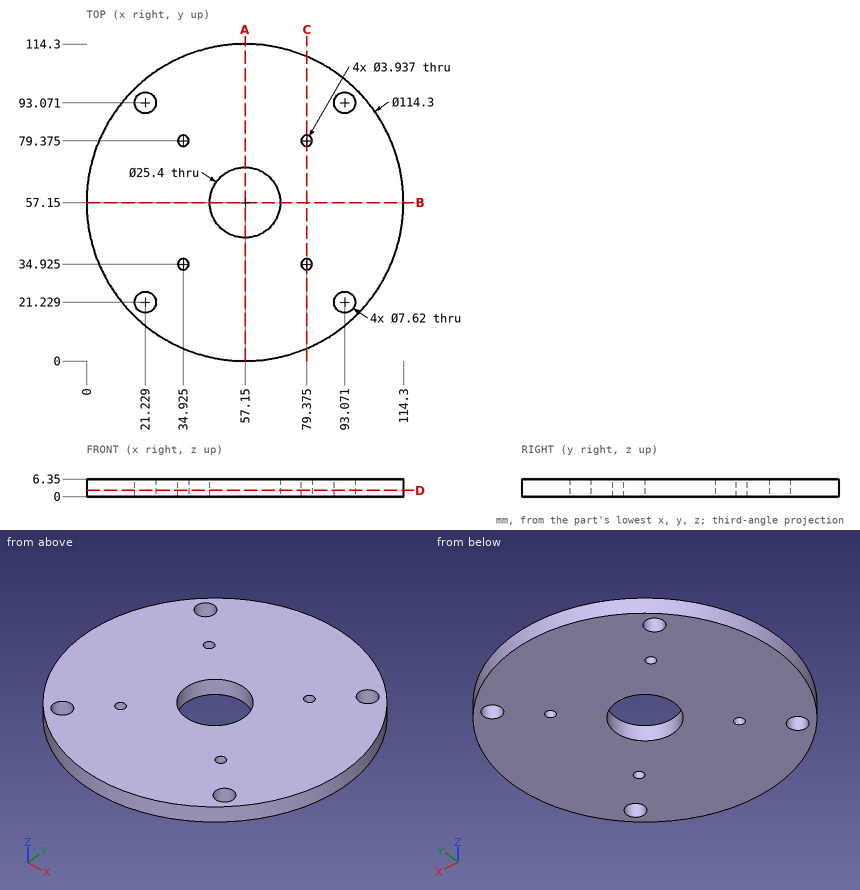
Design review of the part shown in the three views and the two pictorial views. Dimensions are in mm from the part's minimum x, y and z. Coordinates: 2 decimals unless noted, no trailing zeros. Write each loop counter-clockwise with the first axis right and the second up, starting at its lowest first coordinate (ties: lowest second). Pieces come first, ordered by that corner, then holes.
(1) Add section A-A on x = 57.15. Give the boundary of the cut face in (y, z), then the cut area to 3 significant figures.
(2) For pin 1 Ø12 at (x, y) = (21.23, 21.23) entering from +Z; pin 2 Ø1.5 at (x, z) = (17.5, 1.5) entering from -Y; pin 3 Ø2.5 at (x, y) = (79.375, 79.375) entering from -Z; pin 4 Ø1 at (y, z) = (60.5, 1) entering from +X, all flat-tipped, find the tip position at first contact; note any pin that passes through.
(3) Add section C-C on x = 79.5. Give the boundary of the cut face in (y, z), then the cut area to 3 significant figures.
(4) Wall thickness on probe 1 along X at (y, z) = (36, 1.25); probe 2 along Y at (x, z) = (57.5, 2.5); probe 3 along Y at (x, z) = (95, 5): over which ranges is each line inside the solid? List them lowest first.
(5) Add section D-D on z = 2.25. Count the separate pieces of the cut face and the enclosed holes in it, then the cut area to 3 significant figures.
Answer sheet:
1. outline: (0, 0) - (44.45, 0) - (44.45, 6.35) - (0, 6.35) - close; (69.85, 0) - (114.3, 0) - (114.3, 6.35) - (69.85, 6.35) - close
1. area: 565 mm2
2. pin 1: stops at z = 6.35
2. pin 2: stops at y = 15.28
2. pin 3: passes through
2. pin 4: stops at x = 114.23
3. outline: (4.55, 0) - (32.96, 0) - (32.96, 6.35) - (4.55, 6.35) - close; (36.89, 0) - (77.41, 0) - (77.41, 6.35) - (36.89, 6.35) - close; (81.34, 0) - (109.75, 0) - (109.75, 6.35) - (81.34, 6.35) - close
3. area: 618 mm2
4. probe 1: x = 4.06 to 33.28, 36.57 to 77.73, 81.02 to 110.24
4. probe 2: y = 0 to 44.45, 69.85 to 114.3
4. probe 3: y = 14.33 to 17.94, 24.51 to 89.79, 96.36 to 99.97
5. separate pieces: 1
5. enclosed holes: 9
5. area: 9,520 mm2
